For this review, take the finished solid that the model builds, in its own axes (mm). A direction names the side the tool comes from. Round coordinates to 2 decimals unless told otherwise and drop trailing zeros. Order: outer loops, then holes, each group sorted by start corner. A loop starts at its lowest first (then second) coordinate and runs counter-clockwise, first axis right, second up.
```python
from build123d import *

# Parameters (mm, degrees)
SKETCH1_R           = 4
SKETCH1_R_2         = 12
BOSS_EXTRUDE1_DEPTH = 2.5
FILLET1_R           = 4
CHAMFER1_SIZE       = 1


with BuildPart() as part:
    # Sketch1 → Boss-Extrude1 (new body, symmetric)
    with BuildSketch(Plane(origin=(0, 0, 0), x_dir=(1, 0, 0), z_dir=(0, 1, 0))):
        with BuildLine():
            Line((37, 11), (3.508016814, 17.654852535))
            ThreePointArc((3.508016814, 17.654852535), (0, 18), (-3.508016814, 17.654852535))
            Line((-3.508016814, 17.654852535), (-37, 11))
            ThreePointArc((-37, 11), (-48, 0), (-37, -11))
            Line((-37, -11), (-3.508016814, -17.654852535))
            ThreePointArc((-3.508016814, -17.654852535), (0, -18), (3.508016814, -17.654852535))
            Line((3.508016814, -17.654852535), (37, -11))
            ThreePointArc((37, -11), (48, 0), (37, 11))
        make_face()
        with Locations((37, 0)):
            Circle(SKETCH1_R, mode=Mode.SUBTRACT)
        with Locations((-37, 0)):
            Circle(SKETCH1_R, mode=Mode.SUBTRACT)
        Circle(SKETCH1_R_2, mode=Mode.SUBTRACT)
        with BuildLine():
            Line((-28.954155956, -7.500959513), (-14.744742226, -10.324368102))
            ThreePointArc((-14.744742226, -10.324368102), (-18, 0), (-14.744742226, 10.324368102))
            Line((-14.744742226, 10.324368102), (-28.954155956, 7.500959513))
            ThreePointArc((-28.954155956, 7.500959513), (-26, 0), (-28.954155956, -7.500959513))
        make_face(mode=Mode.SUBTRACT)
        with BuildLine():
            ThreePointArc((14.744742226, 10.324368102), (18, 0), (14.744742226, -10.324368102))
            Line((14.744742226, -10.324368102), (28.954155956, -7.500959513))
            ThreePointArc((28.954155956, -7.500959513), (26, 0), (28.954155956, 7.500959513))
            Line((28.954155956, 7.500959513), (14.744742226, 10.324368102))
        make_face(mode=Mode.SUBTRACT)
    extrude(amount=BOSS_EXTRUDE1_DEPTH, both=True)

    # Fillet1
    fillet1_edges = [part.edges().sort_by_distance(p)[0] for p in [
        (14.744742226, 0, 10.324368102),
        (28.954155956, 0, 7.500959513),
        (28.954155956, 0, -7.500959513),
        (14.744742226, 0, -10.324368102),
        (-14.744742226, 0, 10.324368102),
        (-14.744742226, 0, -10.324368102),
        (-28.954155956, 0, -7.500959513),
        (-28.954155956, 0, 7.500959513),
    ]]
    fillet(fillet1_edges, radius=FILLET1_R)

    # Chamfer1
    chamfer1_edges = [part.edges().sort_by_distance(p)[0] for p in [
        (-41, -2.5, 0),
        (33, -2.5, 0),
    ]]
    chamfer(chamfer1_edges, length=CHAMFER1_SIZE)


solid = part.part
```
Q1. Take a section at C-C, the plane z = -7.5. State the section outline as (x, y) points, plus the area to 3 significant figures.
Q2. Tool access review of faces 4 (the face through (-26, 0, 0)), 5 (the face through (-20.02, 0.035, -14.374)): name each direction out of +Z, -Z, +X, -X, +Y, -Y from which nothing blocks a thin tool from reaching the whole face with its end or side.
Q3. Clearance check with flat-ended pins moving along their axes: pin 1 (13 mm diameter, centred on x = 37, z = 0, fed in from +Y); pin 2 (3 mm diameter, centred on y = 0, z = -10.5, fed in from +X); pin 3 (2 mm diameter, centred on x = -24.5, y = 1, fed in from +Z). State where each tip first meets the part, or that it passes through.
Q4. Take a section at B-B, the plane z = 0. State the section outline as (x, y) points, plus the area to 3 significant figures.
Q5. Take a section at D-D, the plane x = -30.5. State the section outline as (y, z) points, plus the area to 3 significant figures.
Q6. Wall thickness on line 1 (Z direction, x = -37, y = -0.15); line 2 (X direction, y = 2, z = 8); line 3 (Z direction, x = 35.5, y = 1.55): over which ranges is each line inside the solid? List them lowest first.
Q7. Take a section at A-A, the plane x = 0. State the section outline as (y, z) points, plus the area to 3 significant figures.
Q8. Mouldability with a two-part tool opening along Z and no side actions: class faces 1 (the face through (26.17, 0.04, -6.72)), 2 (the face through (-20.49, 0.04, 14.28)), 3 (the face through (48, 0, 0)) as +Z half, -Z half, draft (parallel to the pull), parting line (faces both ways), or undercut.
Working result:
1. outline: (-45.05, -2.5) - (-25.56, -2.5) - (-25.56, 2.5) - (-45.05, 2.5) - close; (-18.39, -2.5) - (-9.37, -2.5) - (-9.37, 2.5) - (-18.39, 2.5) - close; (9.37, -2.5) - (18.39, -2.5) - (18.39, 2.5) - (9.37, 2.5) - close; (25.56, -2.5) - (45.05, -2.5) - (45.05, 2.5) - (25.56, 2.5) - close
1. area: 285 mm2
2. face 4: +Y, -Y
2. face 5: -Z, -X, +Y, -Y
3. pin 1: stops at y = 2.5
3. pin 2: stops at x = 43.32
3. pin 3: stops at z = 13.68
4. outline: (-48, -2.5) - (-42, -2.5) - (-41, -1.5) - (-41, 2.5) - (-48, 2.5) - close; (-33, -1.5) - (-32, -2.5) - (-26, -2.5) - (-26, 2.5) - (-33, 2.5) - close; (-18, -2.5) - (-12, -2.5) - (-12, 2.5) - (-18, 2.5) - close; (12, -2.5) - (18, -2.5) - (18, 2.5) - (12, 2.5) - close; (26, -2.5) - (32, -2.5) - (33, -1.5) - (33, 2.5) - (26, 2.5) - close; (41, -1.5) - (42, -2.5) - (48, -2.5) - (48, 2.5) - (41, 2.5) - close
4. area: 198 mm2
5. outline: (-2.5, -12.29) - (2.5, -12.29) - (2.5, 12.29) - (-2.5, 12.29) - close
5. area: 123 mm2
6. line 1: z = -11 to -4, 4 to 11
6. line 2: x = -44.55 to -24.94, -18.9 to -8.94, 8.94 to 18.9, 24.94 to 44.55
6. line 3: z = -11.3 to -3.71, 3.71 to 11.3
7. outline: (-2.5, -18) - (2.5, -18) - (2.5, -12) - (-2.5, -12) - close; (-2.5, 12) - (2.5, 12) - (2.5, 18) - (-2.5, 18) - close
7. area: 60.0 mm2
8. face 1: undercut
8. face 2: +Z half
8. face 3: parting line
